The listing builds one solid part. Answer for the finished solid, in the listing's coordinates (mm). Face numbers are marked on the shaded views. Round coordinates to 2 decimals unless told otherwise and drop trailing zeros. Loops run counter-clockwise (first coordinate to the right, second up) from the corner with the lowest first, then second, coordinate; pieces in that order, holes last. Notation, with made-up numbers: (-35, 19) -> (-29, 19) arc R14 ccw to (-29, 41) -> close; hole circle Ø5 at (74.5, 20.25). An arc over 180 degrees is marked (long way). Use a Markdown table: item, result. Add a question column.
Q1. Given pin 1 Ø3 at (y, z) = (57.5, 36.5) entering from +X; pin 2 Ø2 at (y, z) = (97.5, -33) entering from -X; pin 3 Ø5 at (x, z) = (0.5, 31.5) entering from +Y, each flat-ended and moving along its own axis, determine where each tip first touches the part or whether it passes through.
Q2. Consider line 1 (Z direction, x = 0, y = 84); line 2 (Z direction, x = 0, y = 18.5). Determine where each line is inside the solid, lowest interval first.
Q3. For a pull along X with two mould halves and no side action, classify the marked faces 1, 2 and 3 as released by +X, released by -X, zero draft, split by the parting line, or undercut.
Q4. Section C-C on y = 116.5 is taken. Give the vertices of the cut face in (x, z), then the cut area to 3 significant figures.
Autodesk Inventor part; units mm, degrees
ref_plane "YZ Plane" through (0, 0, 0) normal (1, 0, 0) x (0, 1, 0)
ref_plane "XZ Plane" through (0, 0, 0) normal (0, 1, 0) x (-1, 0, 0)
ref_plane "XY Plane" through (0, 0, 0) normal (0, 0, 1) x (1, 0, 0)
sketch "Sketch1" plane through (0, 0, 0) normal (0, 0, 1) x (1, 0, 0)
  line L0 (0, 0) -> (50, 0)
  line L1 (50, 0) -> (50, 20)
  line L2 (0, 0) -> (0, 125)
  line L3 (0, 125) -> (50, 125)
  line L4 (50, 125) -> (50, 20)
  dimension "d15" = 125
revolve "Revolution1" add sketch "Sketch1" angle 360 about axis through (0, 0, 0) along (0, 1, 0)
shell "Shell1" thickness 1 removed faces 1 at (-6.8644, 125, 10.9394)
sketch "Sketch2" plane through (0, 1, 0) normal (0, 1, 0) x (1, 0, 0)
  circle A0 centre (0, 0) radius 49
  circle A1 centre (0, 0) radius 49
extrude "Extrusion1" add sketch "Sketch2" along normal blind 39
fillet "Fillet1" radius 0.5 3 edges at (-50, 125, 0) (-49, 125, 0) (-50, 0, 0)
sketch "Sketch3" plane through (0, 0, 0) normal (0, -1, 0) x (1, 0, 0)
  circle A0 centre (0, 0) radius 49.5
  circle A1 centre (0, 0) radius 20
extrude "Extrusion2" cut sketch "Sketch3" against normal blind 29 contours A1
fillet "Fillet2" radius 15 1 edges at (-20, 0, 0)
fillet "Fillet3" radius 5 1 edges at (-20, 29, 0)
properties part number "Visk"
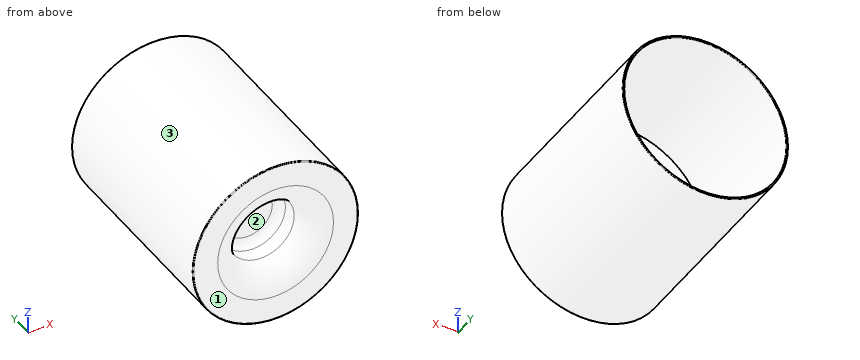
Checked values:
| question | item | result |
|---|---|---|
| 1 | pin 1 | stops at x = 35.71 |
| 1 | pin 2 | stops at x = -38.42 |
| 1 | pin 3 | stops at y = 40 |
| 2 | line 1 | z = -50 to -49, 49 to 50 |
| 2 | line 2 | z = -50 to -20, 20 to 50 |
| 3 | face 1 | zero draft |
| 3 | face 2 | undercut |
| 3 | face 3 | split by the parting line |
| 4 | outline | circle Ø100 at (0, 0); hole circle Ø98 at (0, 0) |
| 4 | area | 311 mm2 |
